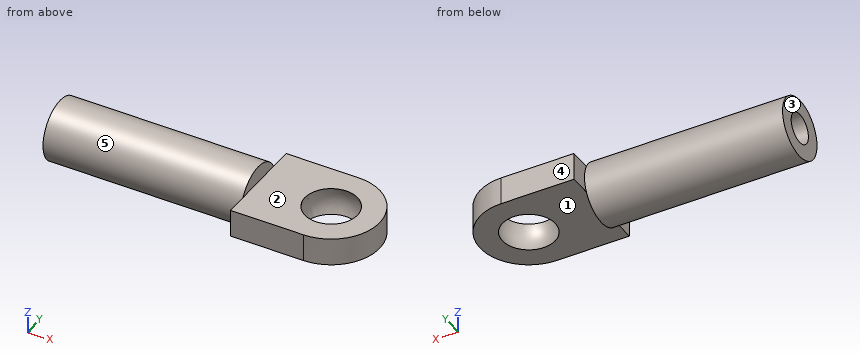
from build123d import *

# Parameters (mm, degrees)
EXTRUDE1_DEPTH      = 1.1049
EXTRUDE1_DEPTH_BACK = 1.1049
SKETCH2_R           = 2.413
EXTRUDE2_DEPTH      = 15.875
SKETCH3_R           = 1.2065
EXTRUDE3_DEPTH      = 14.859


with BuildPart() as part:
    # Sketch1 → Extrude1 (new body, two sides)
    with BuildSketch(Plane.XY) as extrude1_sk:
        with BuildLine():
            Line((0, 3.8862), (-5.842, 3.8862))
            Line((-5.842, 3.8862), (-5.842, -3.8862))
            Line((-5.842, -3.8862), (0, -3.8862))
            ThreePointArc((0, -3.8862), (3.8862, 0), (0, 3.8862))
        make_face()
    extrude(amount=EXTRUDE1_DEPTH)
    extrude(extrude1_sk.sketch, amount=-EXTRUDE1_DEPTH_BACK)

    # Sketch2 → Extrude2 (add)
    with BuildSketch(Plane.ZY.offset(5.842)):
        Circle(SKETCH2_R)
    extrude(amount=EXTRUDE2_DEPTH)

    # Sketch3 → Extrude3 (cut)
    with BuildSketch(Plane.ZY.offset(21.717)):
        Circle(SKETCH3_R)
    extrude(amount=-EXTRUDE3_DEPTH, mode=Mode.SUBTRACT)

    # Sketch6 → Cut-Revolve1 (revolve, cut)
    with BuildSketch(Plane.XY):
        with BuildLine():
            Line((0, -2.38125), (0, 2.38125))
            ThreePointArc((0, 2.38125), (-2.38125, 0), (0, -2.38125))
        make_face()
    revolve(axis=Axis((0, -2.38125, 0), (0, 1, 0)), mode=Mode.SUBTRACT)


solid = part.part
Verification items for the finished model (mm, model axes). Face numbers are marked on the shaded views. A direction names the side the tool comes from. Coordinates: 2 decimals unless noted, no trailing zeros. Order: outer loops, then holes, each group sorted by start corner. A loop starts at its lowest first (then second) coordinate and runs counter-clockwise, first axis right, second up.
Item 1: Section check C-C, the plane x = -1. Enter the section's corners in (y, z).
Filled in:
outline: (-3.89, -1.1) - (-1.86, -1.1) arc R2.16 cw to (-1.86, 1.1) - (-3.89, 1.1) - close; (1.86, -1.1) - (3.89, -1.1) - (3.89, 1.1) - (1.86, 1.1) arc R2.16 cw to start
Item 2: Access from +Z, -Z, +X, -X, +Y, -Y to the whole of each face (thin tool, end or side, straight path). Record for the marked faces 1, 2, 3, 4 and 5.
Filled in:
face 1: -Z, +X, +Y, -Y
face 2: +Z, +X, +Y, -Y
face 3: +Z, -Z, -X, +Y, -Y
face 4: +Z, -Z, +X, -X, +Y
face 5: -X
Item 3: Section check B-B, the plane z = 0. Enter the section's corners in (x, y), then the cut area to 3 significant figures.
Filled in:
outline: (-21.72, -2.41) - (-5.84, -2.41) - (-5.84, -3.89) - (0, -3.89) arc R3.89 ccw to (0, 3.89) - (-5.84, 3.89) - (-5.84, 2.41) - (-21.72, 2.41) - (-21.72, 1.21) - (-6.86, 1.21) - (-6.86, -1.21) - (-21.72, -1.21) - close; hole circle Ø4.76 at (0, 0)
area: 92.1 mm2
Item 4: Section check D-D, the plane x = -19.75. Enter the section's corners in (y, z), then the cut area to 3 significant figures.
Filled in:
outline: circle Ø4.83 at (0, 0); hole circle Ø2.41 at (0, 0)
area: 13.7 mm2
Item 5: Depth check by flat-ended pin: pin 1 (1 mm diameter, centred on y = 0, z = -0.5, fed in from -X); pin 2 (0.9 mm diameter, centred on y = -3, z = 0, fed in from -X); pin 3 (4 mm diameter, centred on x = 0.5, y = 1, fed in from -Z); pin 4 (1.2 mm diameter, centred on y = 0.5, z = 0.5, fed in from -X). Enter the tip coordinate at first touch or a pass-through.
Filled in:
pin 1: stops at x = -6.86
pin 2: stops at x = -5.84
pin 3: stops at z = -1.1
pin 4: stops at x = -21.72
Item 6: Section check A-A, the plane y = 1.75. Enter the section's corners in (x, z), then the cut area to 3 significant figures.
Filled in:
outline: (-21.72, -1.66) - (-5.84, -1.66) - (-5.84, -1.1) - (-1.18, -1.1) arc R1.61 cw to (-1.18, 1.1) - (-5.84, 1.1) - (-5.84, 1.66) - (-21.72, 1.66) - close; (1.18, -1.1) - (3.47, -1.1) - (3.47, 1.1) - (1.18, 1.1) arc R1.61 cw to start
area: 66.8 mm2
Item 7: Material ranges on L1, parallel to Y at x = -16.5, z = 0; L2, parallel to X at y = -0.75, z = -1.9; L3, parallel to X at y = 1.25, z = -0.25, recorded low to high.
Filled in:
L1: y = -2.41 to -1.21, 1.21 to 2.41
L2: x = -21.72 to -5.84
L3: x = -21.72 to -2.01, 2.01 to 3.68
